```python
from build123d import *

# Parameters (mm, degrees)
SKETCH1_R           = 7.5
BOSS_EXTRUDE1_DEPTH = 10
SKETCH2_R           = 12.5
BOSS_EXTRUDE2_DEPTH = 2
BOSS_EXTRUDE3_START = -2
SKETCH3_R           = 12.5
BOSS_EXTRUDE3_DEPTH = 2
SKETCH4_R           = 2
BOSS_EXTRUDE4_DEPTH = 40
BOSS_EXTRUDE5_START = 40
SKETCH5_R           = 2
BOSS_EXTRUDE5_DEPTH = 40


with BuildPart() as part:
    # Sketch1 → Boss-Extrude1 (new body)
    with BuildSketch(Plane.XY):
        Circle(SKETCH1_R)
    extrude(amount=BOSS_EXTRUDE1_DEPTH)

    # Sketch2 → Boss-Extrude2 (add)
    with BuildSketch(Plane(origin=(0, 0, 0), x_dir=(-1, 0, 0), z_dir=(0, 0, -1))):
        Circle(SKETCH2_R)
    extrude(amount=-BOSS_EXTRUDE2_DEPTH)

    # Sketch3 → Boss-Extrude3 (add)
    with BuildSketch(Plane.XY.offset(10).offset(BOSS_EXTRUDE3_START)):
        with Locations(Location((0, 0, 0), (0, 0, 180))):
            Circle(SKETCH3_R)
    extrude(amount=BOSS_EXTRUDE3_DEPTH)

    # Sketch4 → Boss-Extrude4 (add)
    with BuildSketch(Plane.XY.offset(10)):
        Circle(SKETCH4_R)
    extrude(amount=BOSS_EXTRUDE4_DEPTH)

    # Sketch5 → Boss-Extrude5 (add)
    with BuildSketch(Plane(origin=(0, 0, 0), x_dir=(-1, 0, 0), z_dir=(0, 0, -1)).offset(BOSS_EXTRUDE5_START)):
        with Locations(Location((0, 0, 0), (0, 0, 180))):
            Circle(SKETCH5_R)
    extrude(amount=-BOSS_EXTRUDE5_DEPTH)


solid = part.part
```
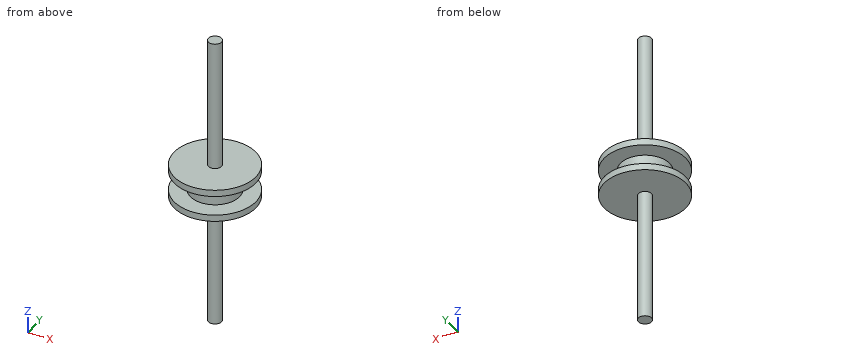
Work out the finished part from the listing and answer in its coordinate system (mm). Coordinates: 2 decimals unless noted, no trailing zeros. Write each loop counter-clockwise with the first axis right and the second up, starting at its lowest first coordinate (ties: lowest second). Pieces come first, ordered by that corner, then holes.
Q1. Find the intervals of material crossed by line 1 (Z direction, x = -5, y = 7); line 2 (Z direction, x = -1, y = -4.5); line 3 (Y direction, x = -0.25, z = -19), in increasing order.
Q2. A cutting plane is placed at C-C, the plane x = 0. Give the vertices of the cut face in (y, z), then the cut area to 3 significant figures.
Q3. Each of these flat-tipped pins is pushed along its axis until it touches: pin 1 Ø4 at (y, z) = (3, -3) entering from +X; pin 2 Ø12.5 at (x, y) = (-6, 2) entering from +Z; pin 3 Ø1 at (y, z) = (4, 5.5) entering from -X; pin 4 Ø5 at (x, y) = (9.5, 7.5) entering from -Z. Where does it stop, or does it pass through?
Q4. A cutting plane is placed at B-B, the plane y = 9.5. Give the vertices of the cut face in (x, z).
Q5. A cutting plane is placed at A-A, the plane x = 10.75. Give the vertices of the cut face in (y, z).
Findings below:
1. line 1: z = 0 to 2, 8 to 10
1. line 2: z = 0 to 10
1. line 3: y = -1.98 to 1.98
2. outline: (-12.5, 0) - (-2, 0) - (-2, -40) - (2, -40) - (2, 0) - (12.5, 0) - (12.5, 2) - (7.5, 2) - (7.5, 8) - (12.5, 8) - (12.5, 10) - (2, 10) - (2, 50) - (-2, 50) - (-2, 10) - (-12.5, 10) - (-12.5, 8) - (-7.5, 8) - (-7.5, 2) - (-12.5, 2) - close
2. area: 510 mm2
3. pin 1: stops at x = 1.73
3. pin 2: stops at z = 50
3. pin 3: stops at x = -6.63
3. pin 4: stops at z = 0
4. outline: (-8.12, 0) - (8.12, 0) - (8.12, 2) - (-8.12, 2) - close; (-8.12, 8) - (8.12, 8) - (8.12, 10) - (-8.12, 10) - close
5. outline: (-6.38, 0) - (6.38, 0) - (6.38, 2) - (-6.38, 2) - close; (-6.38, 8) - (6.38, 8) - (6.38, 10) - (-6.38, 10) - close
